Autodesk Inventor part; units mm, degrees
ref_plane "YZ Plane" through (0, 0, 0) normal (1, 0, 0) x (0, 1, 0)
ref_plane "XZ Plane" through (0, 0, 0) normal (0, 1, 0) x (-1, 0, 0)
ref_plane "XY Plane" through (0, 0, 0) normal (0, 0, 1) x (1, 0, 0)
sketch "Sketch1" plane through (0, 0, 0) normal (0, 0, 1) x (1, 0, 0)
  line L0 (0, 40) -> (0, 0)
  line L1 (0, 40) -> (3.5, 40)
  line L2 (3.5, 40) -> (3.5, 0)
  line L3 (0, 0) -> (3.5, 0)
  line L4 (0, 57) -> (3.5, 57)
  line L5 (3.5, 53) -> (0, 53)
  line L6 (0, -13) -> (3.5, -13)
  line L7 (3.5, -17) -> (0, -17)
  line L8 (0, -30) -> (0, -70)
  line L9 (0, -30) -> (3.5, -30)
  line L10 (3.5, -30) -> (3.5, -70)
  line L11 (0, -70) -> (3.5, -70)
  line L12 (0, -100) -> (0, -140)
  line L13 (3.5, -100) -> (3.5, -140)
  line L14 (0, -100) -> (3.5, -100)
  line L15 (0, -140) -> (3.5, -140)
  line L16 (0, -153) -> (3.5, -153)
  line L17 (3.5, -157) -> (0, -157)
  line L18 (263.5, 57.0001) -> (267, 57.0001)
  line L19 (267, 53.0001) -> (263.5, 53.0001)
  line L20 (263.5, 40.0001) -> (267, 40.0001)
  line L21 (263.5, 40.0001) -> (263.5, 0.0001)
  line L22 (267, 40.0001) -> (267, 0.0001)
  line L23 (263.5, 0.0001) -> (267, 0.0001)
  line L24 (263.5, -12.9999) -> (267, -12.9999)
  line L25 (267, -16.9999) -> (263.5, -16.9999)
  line L26 (263.5, -29.9999) -> (267, -29.9999)
  line L27 (263.5, -29.9999) -> (263.5, -69.9999)
  line L28 (267, -29.9999) -> (267, -69.9999)
  line L29 (263.5, -69.9999) -> (267, -69.9999)
  line L30 (263.5, -99.9999) -> (263.5, -139.9999)
  line L31 (263.5, -99.9999) -> (267, -99.9999)
  line L32 (267, -99.9999) -> (267, -139.9999)
  line L33 (263.5, -139.9999) -> (267, -139.9999)
  line L34 (263.5, -152.9999) -> (267, -152.9999)
  line L35 (267, -156.9999) -> (263.5, -156.9999)
  line L36 (23.5, -149.9999) -> (23.5, -144.9999)
  line L37 (27.5, -144.9999) -> (27.5, -149.9999)
  line L38 (37.5, -144.9999) -> (37.5, -149.9999)
  line L39 (57.5, -144.9999) -> (57.5, -149.9999)
  line L40 (67.5, -149.9999) -> (67.5, -144.9999)
  line L41 (71.5, -144.9999) -> (71.5, -149.9999)
  line L42 (37.5, -144.9999) -> (57.5, -144.9999)
  line L43 (57.5, -149.9999) -> (37.5, -149.9999)
  line L44 (103.5, -144.9999) -> (103.5, -149.9999)
  line L45 (103.5, -144.9999) -> (163.5, -144.9999)
  line L46 (163.5, -149.9999) -> (103.5, -149.9999)
  line L47 (163.5, -144.9999) -> (163.5, -149.9999)
  line L48 (195.5, -149.9999) -> (195.5, -144.9999)
  line L49 (199.5, -144.9999) -> (199.5, -149.9999)
  line L50 (209.5, -144.9999) -> (209.5, -149.9999)
  line L51 (229.5, -144.9999) -> (229.5, -149.9999)
  line L52 (209.5, -144.9999) -> (229.5, -144.9999)
  line L53 (229.5, -149.9999) -> (209.5, -149.9999)
  line L54 (239.5, -149.9999) -> (239.5, -144.9999)
  line L55 (243.5, -144.9999) -> (243.5, -149.9999)
  line L56 (253.5, -84.9999) -> (253.5, -89.9999)
  line L57 (249.5, -89.9999) -> (249.5, -84.9999)
  line L58 (239.5, -84.9999) -> (239.5, -89.9999)
  line L59 (239.5, -84.9999) -> (219.5, -84.9999)
  line L60 (219.5, -84.9999) -> (219.5, -89.9999)
  line L61 (239.5, -89.9999) -> (219.5, -89.9999)
  line L62 (205.5, -89.9999) -> (205.5, -84.9999)
  line L63 (209.5, -84.9999) -> (209.5, -89.9999)
  line L64 (103.5, -84.9999) -> (163.5, -84.9999)
  line L65 (163.5, -89.9999) -> (103.5, -89.9999)
  line L66 (163.5, -84.9999) -> (163.5, -89.9999)
  line L67 (103.5, -84.9999) -> (103.5, -89.9999)
  line L68 (57.5, -89.9999) -> (57.5, -84.9999)
  line L69 (61.5, -84.9999) -> (61.5, -89.9999)
  line L70 (47.5, -84.9999) -> (47.5, -89.9999)
  line L71 (27.5, -84.9999) -> (47.5, -84.9999)
  line L72 (47.5, -89.9999) -> (27.5, -89.9999)
  line L73 (27.5, -84.9999) -> (27.5, -89.9999)
  line L74 (13.5, -89.9999) -> (13.5, -84.9999)
  line L75 (17.5, -84.9999) -> (17.5, -89.9999)
  line L76 (-15, 82) -> (-15, -161.9999)
  arc A0 (-7, 90) -> (-15, 82) centre (-7, 82) ccw
  line L77 (274, 90) -> (-7, 90)
  arc A1 (282, 82) -> (274, 90) centre (274, 82) ccw
  line L78 (282, -161.9999) -> (282, 82)
  arc A2 (-15, -161.9999) -> (-7, -169.9999) centre (-7, -161.9999) ccw
  line L79 (-7, -169.9999) -> (274, -169.9999)
  arc A3 (274, -169.9999) -> (282, -161.9999) centre (274, -161.9999) ccw
  line L80 (1.75, 57) -> (1.75, 53)
  line L81 (1.75, -13) -> (1.75, -17)
  line L82 (1.75, -153) -> (1.75, -157)
  line L83 (23.5, -147.4999) -> (27.5, -147.4999)
  line L84 (67.5, -147.4999) -> (71.5, -147.4999)
  line L85 (195.5, -147.4999) -> (199.5, -147.4999)
  line L86 (239.5, -147.4999) -> (243.5, -147.4999)
  line L87 (265.25, -156.9999) -> (265.25, -152.9999)
  line L88 (13.5, -87.4999) -> (17.5, -87.4999)
  line L89 (57.5, -87.4999) -> (61.5, -87.4999)
  line L90 (205.5, -87.4999) -> (209.5, -87.4999)
  line L91 (249.5, -87.4999) -> (253.5, -87.4999)
  line L92 (265.25, -16.9999) -> (265.25, -12.9999)
  line L93 (265.25, 53.0001) -> (265.25, 57.0001)
  circle A4 centre (1.75, 55) radius 2
  circle A5 centre (1.75, -15) radius 2
  circle A6 centre (1.75, -155) radius 2
  circle A7 centre (25.5, -147.4999) radius 2
  circle A8 centre (69.5, -147.4999) radius 2
  circle A9 centre (197.5, -147.4999) radius 2
  circle A10 centre (241.5, -147.4999) radius 2
  circle A11 centre (265.25, -154.9999) radius 2
  circle A12 centre (15.5, -87.4999) radius 2
  circle A13 centre (59.5, -87.4999) radius 2
  circle A14 centre (207.5, -87.4999) radius 2
  circle A15 centre (251.5, -87.4999) radius 2
  circle A16 centre (265.25, -14.9999) radius 2
  circle A17 centre (265.25, 55.0001) radius 2
extrude "Extrusion1" add sketch "Sketch1" along normal blind 3.5
sketch "Sketch2" plane through (0, 0, 3.5) normal (0, 0, 1) x (1, 0, 0)
  line L0 (163.5, -84.9999) -> (163.5, -89.9999) construction
  line L1 (163.5, -89.9999) -> (103.5, -89.9999) construction
  line L2 (103.5, -89.9999) -> (103.5, -84.9999) construction
  line L3 (103.5, -84.9999) -> (163.5, -84.9999) construction
  line L4 (103.5, -144.9999) -> (163.5, -144.9999) construction
  line L5 (163.5, -144.9999) -> (163.5, -149.9999) construction
  line L6 (163.5, -149.9999) -> (103.5, -149.9999) construction
  line L7 (103.5, -149.9999) -> (103.5, -144.9999) construction
  line L8 (263.5, -99.9999) -> (267, -99.9999) construction
  line L9 (267, -99.9999) -> (267, -139.9999) construction
  line L10 (267, -139.9999) -> (263.5, -139.9999) construction
  line L11 (263.5, -139.9999) -> (263.5, -99.9999) construction
  line L12 (267, -29.9999) -> (267, -69.9999) construction
  line L13 (267, -69.9999) -> (263.5, -69.9999) construction
  line L14 (263.5, -69.9999) -> (263.5, -29.9999) construction
  line L15 (263.5, -29.9999) -> (267, -29.9999) construction
  line L16 (267, 40.0001) -> (267, 0.0001) construction
  line L17 (267, 0.0001) -> (263.5, 0.0001) construction
  line L18 (263.5, 0.0001) -> (263.5, 40.0001) construction
  line L19 (263.5, 40.0001) -> (267, 40.0001) construction
  line L20 (0, -100) -> (3.5, -100) construction
  line L21 (3.5, -100) -> (3.5, -140) construction
  line L22 (3.5, -140) -> (0, -140) construction
  line L23 (0, -140) -> (0, -100) construction
  line L24 (0, -30) -> (3.5, -30) construction
  line L25 (3.5, -30) -> (3.5, -70) construction
  line L26 (3.5, -70) -> (0, -70) construction
  line L27 (0, -70) -> (0, -30) construction
  line L28 (0, 40) -> (3.5, 40) construction
  line L29 (3.5, 40) -> (3.5, 0) construction
  line L30 (3.5, 0) -> (0, 0) construction
  line L31 (0, 0) -> (0, 40) construction
  line L32 (47.5, -89.9999) -> (27.5, -89.9999) construction
  line L33 (27.5, -89.9999) -> (27.5, -84.9999) construction
  line L34 (27.5, -84.9999) -> (47.5, -84.9999) construction
  line L35 (47.5, -84.9999) -> (47.5, -89.9999) construction
  line L36 (239.5, -89.9999) -> (219.5, -89.9999) construction
  line L37 (219.5, -89.9999) -> (219.5, -84.9999) construction
  line L38 (219.5, -84.9999) -> (239.5, -84.9999) construction
  line L39 (239.5, -84.9999) -> (239.5, -89.9999) construction
  line L40 (209.5, -144.9999) -> (229.5, -144.9999) construction
  line L41 (229.5, -144.9999) -> (229.5, -149.9999) construction
  line L42 (229.5, -149.9999) -> (209.5, -149.9999) construction
  line L43 (209.5, -149.9999) -> (209.5, -144.9999) construction
  line L44 (37.5, -144.9999) -> (57.5, -144.9999) construction
  line L45 (57.5, -144.9999) -> (57.5, -149.9999) construction
  line L46 (57.5, -149.9999) -> (37.5, -149.9999) construction
  line L47 (37.5, -149.9999) -> (37.5, -144.9999) construction
  circle A0 centre (265.25, 55.0001) radius 2 construction
  circle A1 centre (265.25, -14.9999) radius 2 construction
  circle A2 centre (251.5, -87.4999) radius 2 construction
  circle A3 centre (207.5, -87.4999) radius 2 construction
  circle A4 centre (59.5, -87.4999) radius 2 construction
  circle A5 centre (15.5, -87.4999) radius 2 construction
  circle A6 centre (265.25, -154.9999) radius 2 construction
  circle A7 centre (241.5, -147.4999) radius 2 construction
  circle A8 centre (197.5, -147.4999) radius 2 construction
  circle A9 centre (69.5, -147.4999) radius 2 construction
  circle A10 centre (25.5, -147.4999) radius 2 construction
  circle A11 centre (1.75, -155) radius 2 construction
  circle A12 centre (1.75, -15) radius 2 construction
  circle A13 centre (1.75, 55) radius 2 construction
  line L48 (-15, 82) -> (-15, -161.9999) construction
  arc A14 (-15, -161.9999) -> (-7, -169.9999) centre (-7, -161.9999) ccw construction
  line L49 (-7, -169.9999) -> (274, -169.9999) construction
  arc A15 (274, -169.9999) -> (282, -161.9999) centre (274, -161.9999) ccw construction
  line L50 (282, -161.9999) -> (282, 82) construction
  arc A16 (282, 82) -> (274, 90) centre (274, 82) ccw construction
  line L51 (274, 90) -> (-7, 90) construction
  arc A17 (-7, 90) -> (-15, 82) centre (-7, 82) ccw construction
  line L52 (-15, 82) -> (-15, 90) construction
  line L53 (-15, 90) -> (-7, 90) construction
  line L54 (-15.8616, 90) -> (7.6384, 90) construction
  line L55 (7.6384, 90) -> (7.6384, 73.5) construction
  line L56 (7.6384, 73.5) -> (-15.8616, 73.5) construction
  line L57 (-15.8616, 73.5) -> (-15.8616, 90) construction
  line L58 (7.6384, 73.5) -> (257.6384, 73.5)
  line L59 (257.6384, 73.5) -> (257.6384, 70)
  line L60 (257.6384, 70) -> (7.6384, 70)
  line L61 (7.6384, 70) -> (7.6384, 73.5)
  dimension "d2" = 23.5
  dimension "d3" = 16.5
  dimension "d4" = 250
  dimension "d5" = 3.5
extrude "Extrusion2" cut sketch "Sketch2" against normal blind 3.5
properties part number "Tapa_Trasera"
Geometry check sheet. Reference: the model listing, model coordinates, mm. Coordinates: 2 decimals unless noted, no trailing zeros. Order: outer loops, then holes, each group sorted by start corner. A loop starts at its lowest first (then second) coordinate and runs counter-clockwise, first axis right, second up. Notation, with made-up numbers: (57, 19.5) - (101, 19.5) arc R20 ccw to (101, 48.5) - close; hole circle Ø7 at (3.25, 84.5). An arc over 180 degrees is marked (long way). Answer as a JSON object with one key per item and string values. Group by question number.
Item 1: Sectioned sample at B-B, the plane z = 1.2. Give the number of separate pieces and of enclosed holes in the cut face, and give its area (3 significant figures).
Item 2: Scan lines: probe 1 along X at (y, z) = (-64.5, 2.45); probe 2 along Y at (x, z) = (111, 2.9); probe 3 along X at (y, z) = (-155, 2.75). Record each from-to range of solid material in increasing order.
Item 3: Depth check by flat-ended pin: pin 1 Ø2.5 at (x, y) = (265.25, -15) entering from +Z. Enter the tip coordinate at first touch or a pass-through.
Item 4: Sectioned sample at A-A, the plane x = 213. Record the cut outline in (y, z), and give its area (3 significant figures).
Resolved:
{
 "1": {"separate pieces": "1", "enclosed holes": "27", "area": "74,300 mm^2"},
 "2": {"probe 1": "-15 to 0, 3.5 to 263.5, 267 to 282", "probe 2": "-170 to -150, -145 to -90, -85 to 70, 73.5 to 90", "probe 3": "-15 to -0.25, 3.75 to 263.25, 267.25 to 282"},
 "3": {"pin 1": "through"},
 "4": {"outline": "(-170, 0) - (-150, 0) - (-150, 3.5) - (-170, 3.5) - close; (-145, 0) - (70, 0) - (70, 3.5) - (-145, 3.5) - close; (73.5, 0) - (90, 0) - (90, 3.5) - (73.5, 3.5) - close", "area": "880 mm^2"}
}
